Read the model definition and answer for the solid it produces. Units are mm, in the model's axes. Coordinates: 2 decimals unless noted, no trailing zeros. One line per item, written item: value. Start each with the question number.
from build123d import *

# Parameters (mm, degrees)
SKETCH5_R          = 65.838775907
SKETCH5_R_2        = 51.340137945
SKETCH5_R_3        = 46.082776278
SKETCH5_R_4        = 36.313221665
SKETCH5_R_5        = 39.620905692
CUT_EXTRUDE1_DEPTH = 54.0000001


with BuildPart() as part:
    # Sketch1 → Loft l4 section 0
    with BuildSketch(Plane(origin=(0, 0, 0), x_dir=(0, 0, -1), z_dir=(1, 0, 0))):
        Polygon((-53, 236), (33, 236), (33, 216), (0, 216), (0, -216), (33, -216), (33, -236), (-53, -236), (-53, -216), (-20, -216), (-20, 216), (-53, 216), align=None)
    # Sketch4 → Loft l4 section 1
    with BuildSketch(Plane(origin=(1250, 0, -1000), x_dir=(0, 0, 1), z_dir=(-1, 0, 0))):
        Polygon((994, 60), (1026, 60), (1026, 40), (1020, 40), (1020, -40), (1026, -40), (1026, -60), (994, -60), (994, -40), (1000, -40), (1000, 40), (994, 40), align=None)
    loft()

    # Sketch5 → Cut-Extrude1 (cut, through all)
    with BuildSketch(Plane.XY.offset(20)):
        with Locations((137.875176339, 0)):
            Circle(SKETCH5_R)
        with Locations((423.461863642, 0)):
            Circle(SKETCH5_R_2)
        with Locations((597.226106195, 0)):
            Circle(SKETCH5_R_3)
        with Locations((825.313339697, 0)):
            Circle(SKETCH5_R_4)
        with Locations((716.202882206, 0)):
            Circle(SKETCH5_R_5)
    extrude(amount=-CUT_EXTRUDE1_DEPTH, mode=Mode.SUBTRACT)


solid = part.part
1. Given pin 1 (4 mm diameter, centred on x = 993.5, z = 12.5, fed in from -Y); pin 2 (4 mm diameter, centred on x = 441.5, z = 26.5, fed in from -Y); pin 3 (1 mm diameter, centred on x = 300, z = -21.5, fed in from +Y), each flat-ended and moving along its own axis, determine where each tip first touches the part or whether it passes through.
2. A cutting plane is placed at A-A on y = 0. Count the separate pieces of the cut face and the enclosed holes in it, then the cut area to 3 significant figures.
3. Find the intervals of material crossed by probe 1 along X at (y, z) = (0, 8.75); probe 2 along Z at (x, y) = (748.5, 53); probe 3 along Y at (x, z) = (266.5, 27.5), in increasing order. Write a range as from..to.
Derived:
1. pin 1: stops at y = -96.4
1. pin 2: stops at y = -174.12
1. pin 3: stops at y = 193.83
2. separate pieces: 6
2. enclosed holes: 0
2. area: 15,400 mm2
3. probe 1: x = 0..72.04, 203.71..372.12, 474.8..551.14, 643.31..676.58, 755.82..789, 861.63..1250
3. probe 2: z = 0..20
3. probe 3: y = -198.48..-178.48, 178.48..198.48
